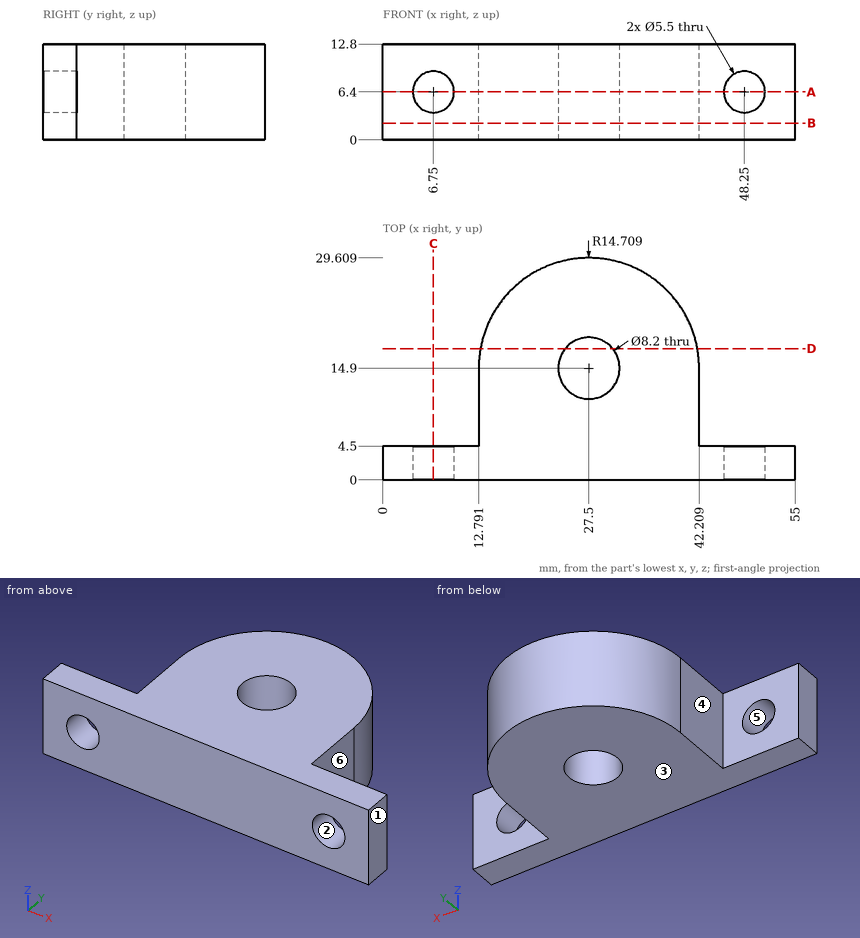
Study the drawing (mm; zero at the part's minimum x, y, z) and answer. A direction names the side the tool comes from. Give positions to 0.01 mm unless a question says otherwise; leave off trailing zeros. Order: outer loops, then holes, each group sorted by start corner. A loop starts at its lowest first (then second) coordinate and runs counter-clockwise, first axis right, second up. Notation, with made-up numbers: (52, -6) - (87, -6) arc R10 cw to (87, 12) - close; hole circle Ø5 at (0, 67.5). An arc over 180 degrees is marked (long way). Answer as CSV lines item,"result". Start each with the question number.
Q1. The part is cut by section B-B (z = 2.25). Write down the section's boundary in (x, y).
Q2. Given pin 1 Ø1.5 at (x, z) = (9.5, 5) entering from +Y; pin 2 Ø3 at (y, z) = (8.5, 9.5) entering from +X, each flat-ended and moving along its own axis, determine where each tip first touches the part or whether it passes through.
Q3. The part is cut by section C-C (x = 6.75). Write down the section's boundary in (y, z).
Q4. For the marked faces 4, 5 and 6, determine the directions among +Z, -Z, +X, -X, +Y, -Y from which every point of the face is accessible in a straight line to the end or side of a thin tool.
Q5. Find the intervals of material crossed by L1, parallel to Z at x = 48.25, y = 3.6; L2, parallel to X at y = 4, z = 7; L3, parallel to Y at x = 39.5, z = 4.75 (1 decimal), in increasing order. Write a range as [from, to].
Q6. The part is cut by section A-A (z = 6.4). Write down the section's boundary in (x, y), then the cut area to 3 significant figures.
Q7. The part is cut by section D-D (y = 17.5). Write down the section's boundary in (x, z).
Q8. The mould has two halves that part along Z. Classify the marked faces 1, 2 and 3: +Z half, -Z half, draft (parallel to the pull), parting line (faces both ways), or undercut.
Check result:
1,outline,"(0, 0) - (55, 0) - (55, 4.5) - (42.21, 4.5) - (42.21, 14.9) arc R14.71 ccw to (12.79, 14.9) - (12.79, 4.5) - (0, 4.5) - close; hole circle Ø8.2 at (27.5, 14.9)"
2,pin 1,"stops at y = 4.5"
2,pin 2,"stops at x = 42.21"
3,outline,"(0, 0) - (4.5, 0) - (4.5, 3.65) - (0, 3.65) - close; (0, 9.15) - (4.5, 9.15) - (4.5, 12.8) - (0, 12.8) - close"
4,face 4,"+Z, -Z, -X, +Y"
4,face 5,"+Y, -Y"
4,face 6,"+Z, -Z, +X, +Y"
5,L1,"z = [0, 3.65], [9.15, 12.8]"
5,L2,"x = [0, 4.07], [9.43, 45.57], [50.93, 55]"
5,L3,"y = [0, 23.4]"
6,outline,"(0, 0) - (4, 0) - (4, 4.5) - (0, 4.5) - close; (9.5, 0) - (45.5, 0) - (45.5, 4.5) - (42.21, 4.5) - (42.21, 14.9) arc R14.71 ccw to (12.79, 14.9) - (12.79, 4.5) - (9.5, 4.5) - close; (51, 0) - (55, 0) - (55, 4.5) - (51, 4.5) - close; hole circle Ø8.2 at (27.5, 14.9)"
6,area,"791 mm²"
7,outline,"(13.02, 0) - (24.33, 0) - (24.33, 12.8) - (13.02, 12.8) - close; (30.67, 0) - (41.98, 0) - (41.98, 12.8) - (30.67, 12.8) - close"
8,face 1,"draft"
8,face 2,"undercut"
8,face 3,"-Z half"
